Read the model definition and answer for the solid it produces. Units are mm, in the model's axes. Face numbers are marked on the shaded views. A direction names the side the tool comes from. Coordinates: 2 decimals unless noted, no trailing zeros. Order: outer loops, then holes, each group sorted by start corner. A loop starts at its lowest first (then second) coordinate and runs counter-clockwise, first axis right, second up. Notation, with made-up numbers: (-37, 68.5) -> (-25, 68.5) arc R14 ccw to (-25, 74.5) -> close; hole circle Ø9 at (82, 9). An arc over 180 degrees is marked (long way). Answer in a Markdown table with one row per item.
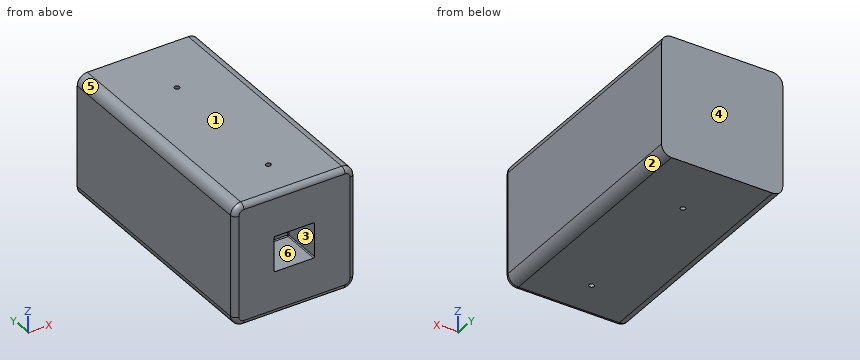
from build123d import *

# Parameters (mm, degrees)
F0_W     = 304.8
F0_H     = 304.8
F0_W_2   = 101.6
F0_H_2   = 88.9
F1_DEPTH = 609.6
F8_DEPTH = 508
F2_R     = 25.4
F3_R     = 12.7
F4_D     = 12.7
F4_DEPTH = 38.1
F4_TIP   = 3.8154649308
F6_D     = 12.7
F6_DEPTH = 38.1
F6_TIP   = 3.8154649308
F7_R     = 2.54


# Not quite as in the source:
# - a feature names something its author has since deleted; it is built from what else it names


with BuildPart() as f1:
    # F0 (on Front) → F1 (new body)
    with BuildSketch(Plane.XZ):
        Rectangle(F0_W, F0_H)
        Rectangle(F0_W_2, F0_H_2, mode=Mode.SUBTRACT)
    extrude(amount=F1_DEPTH)

    # F0 (on Front) → F8 (join)
    with BuildSketch(Plane.XZ):
        Rectangle(F0_W_2, F0_H_2)
    extrude(amount=F8_DEPTH)

    # F2
    f2_edges = [f1.edges().sort_by_distance(p)[0] for p in [
        (152.4, -304.8, -152.4),
        (-152.4, -304.8, -152.4),
        (-152.4, -304.8, 152.4),
        (152.4, -304.8, 152.4),
    ]]
    fillet(f2_edges, radius=F2_R)

    # F3
    f3_edges = [f1.edges().sort_by_distance(p)[0] for p in [
        (152.4, -609.6, 0),
    ]]
    fillet(f3_edges, radius=F3_R)

    # F4
    with Locations(Plane(origin=(0, 0, -152.4), x_dir=(1, 0, 0), z_dir=(0, 0, -1))):
        with Locations((0, 152.4), (0, 508)):
            Hole(F4_D / 2, depth=F4_DEPTH)
            with Locations((0, 0, -(F4_DEPTH + F4_TIP / 2))):  # 118° drill point
                Cone(0, F4_D / 2, F4_TIP, mode=Mode.SUBTRACT)

    # F6
    with Locations(Plane.XY.offset(152.4)):
        with Locations((0, -508), (0, -152.4)):
            Hole(F6_D / 2, depth=F6_DEPTH)
            with Locations((0, 0, -(F6_DEPTH + F6_TIP / 2))):  # 118° drill point
                Cone(0, F6_D / 2, F6_TIP, mode=Mode.SUBTRACT)

    # F7
    f7_edges = [f1.edges().sort_by_distance(p)[0] for p in [
        (-50.8, -558.8, -44.45),
        (-50.8, -558.8, 44.45),
        (50.8, -558.8, 44.45),
        (50.8, -558.8, -44.45),
        (50.8, -508, 0),
        (0, -508, 44.45),
        (-50.8, -508, 0),
        (0, -508, -44.45),
    ]]
    fillet(f7_edges, radius=F7_R)


solid = f1.part
Q1. The part is cut by section A-A (x = 42). Write down the section's boundary in (y, z), then the cut area to 3 significant figures.
Outcome:
| item | result |
|---|---|
| outline | (-609.6, -139.7) arc R12.7 ccw to (-596.9, -152.4) -> (0, -152.4) -> (0, 152.4) -> (-596.9, 152.4) arc R12.7 ccw to (-609.6, 139.7) -> (-609.6, 44.45) -> (-510.54, 44.45) arc R2.54 cw to (-508, 41.91) -> (-508, -41.91) arc R2.54 cw to (-510.54, -44.45) -> (-609.6, -44.45) -> close |
| area | 177,000 mm² |
Q2. For the marked faces 5 and 6, determine the directions among +Z, -Z, +X, -X, +Y, -Y from which every point of the face is accessible in a straight line to the end or side of a thin tool.
Outcome:
| item | result |
|---|---|
| face 5 | +Z, -X, +Y, -Y |
| face 6 | -Y |
Q3. Consider line 1 (Y direction, x = 0, z = -136); line 2 (Z direction, x = -36, y = -574); line 3 (X direction, y = -508, z = -128). Determine where each line is inside the solid, lowest interval first.
Outcome:
| item | result |
|---|---|
| line 1 | -609.6 to -514.35, -501.65 to -158.75, -146.05 to 0 |
| line 2 | -152.4 to -44.45, 44.45 to 152.4 |
| line 3 | -152.38 to -6.35, 6.35 to 152.38 |
Q4. Given pin 1 (25 mm diameter, centred on x = 19, z = -0.5, fed in from -Y); pin 2 (14.5 mm diameter, centred on x = 0, y = -508, fed in from +Z); pin 3 (7.5 mm diameter, centred on x = 0, y = -508, fed in from -Z), each flat-ended and moving along its own axis, determine where each tip first touches the part or whether it passes through.
Outcome:
| item | result |
|---|---|
| pin 1 | y = -508 |
| pin 2 | z = 152.4 |
| pin 3 | z = -112.74 |
Q5. For a pull along Z with two mould halves and no side action, classify the marked faces 1, 2, 3 and 4 as pulls with the +Z half, pulls with the -Z half, needs draft (parallel to the pull), parting line crosses it, or undercut.
Outcome:
| item | result |
|---|---|
| face 1 | pulls with the +Z half |
| face 2 | pulls with the -Z half |
| face 3 | undercut |
| face 4 | needs draft |
